Autodesk Inventor part; units mm, degrees
ref_plane "YZ Plane" through (0, 0, 0) normal (1, 0, 0) x (0, 1, 0)
ref_plane "XZ Plane" through (0, 0, 0) normal (0, 1, 0) x (-1, 0, 0)
ref_plane "XY Plane" through (0, 0, 0) normal (0, 0, 1) x (1, 0, 0)
sketch "Sketch1" plane through (0, 0, 0) normal (0, 0, 1) x (1, 0, 0)
  line L0 (-125.5, -122) -> (125.5, -122)
  line L1 (125.5, -122) -> (125.5, 122)
  line L2 (125.5, 122) -> (-125.5, 122)
  line L3 (-125.5, 122) -> (-125.5, -122)
  line L4 (-125.5, -122) -> (125.5, 122) construction
  line L5 (125.5, -122) -> (-125.5, 122) construction
  line L6 (125.5, 122) -> (47.5, 122)
  line L7 (47.5, 122) -> (47.5, 51)
  line L8 (47.5, 51) -> (125.5, 51)
  line L9 (125.5, 51) -> (125.5, 122)
  point P0 (0, 0)
  point P1 (125.5, 51)
  dimension "d0" = 251
  dimension "d1" = 244
  dimension "d6" = 78
  dimension "d7" = 71
extrude "Extrusion1" add sketch "Sketch1" along normal blind 7 contours L3 L2 L7 L8 L1 L0
sketch "Sketch2" plane through (0, 0, 7) normal (0, 0, 1) x (1, 0, 0)
  line L0 (-100, -100) -> (100, -100)
  line L1 (100, -100) -> (100, 100)
  line L2 (100, 100) -> (-100, 100)
  line L3 (-100, 100) -> (-100, -100)
  line L4 (-100, -100) -> (100, 100) construction
  line L5 (100, -100) -> (-100, 100) construction
  point P0 (0, 0)
  point P1 (0, 0)
  dimension "d4" = 200
  dimension "d5" = 200
sketch "Sketch3" plane through (0, 0, 7) normal (0, 0, 1) x (1, 0, 0)
  line L0 (-85.5721, 144.9839) -> (-125.5, 112)
  line L1 (-125.5, 122) -> (-125.5, -122)
  line L2 (-85.5721, 144.9839) -> (-17.6358, 144.9839) construction
  line L3 (125.5, -122) -> (125.5, 51)
  line L4 (125.5, 51) -> (47.5, 51)
  line L5 (47.5, 51) -> (47.5, 122)
  line L6 (47.5, 122) -> (-125.5, 122)
  line L7 (-125.5, 122) -> (-125.5, -122)
  line L8 (-125.5, -122) -> (125.5, -122)
  point P0 (0, 0)
  point P1 (-113.3947, 122)
  point P2 (-125.5, 122)
  dimension "d9" = 140.44
  dimension "d10" = 10
extrude "Extrusion2" cut sketch "Sketch3" against normal blind 10 contours L0 L1 L6
fillet "Fillet1" radius 5 2 edges at (-113.3947, 122, 3.5) (-125.5, 112, 3.5)
chamfer "Chamfer1" distance 10 angle 45 1 edges at (47.5, 51, 3.5)
sketch "Sketch4" plane through (0, 0, 7) normal (0, 0, 1) x (1, 0, 0)
  line L0 (-125.5, 109.645) -> (-125.5, -122)
  line L1 (125.5, -122) -> (125.5, 51)
  line L2 (-125.5, -122) -> (125.5, -122)
  point P0 (0, 0)
  point P1 (-121, -114.5)
  point P2 (115.5, -114.5)
  point P3 (10, -114.5)
  point P4 (62.75, -114.5)
  dimension "d17" = 4.5
  dimension "d20" = 10
  dimension "d21" = 7.5
  dimension "d42" = 52.75
  dimension "d43" = 52.75
hole "Hole1" at (-121, -114.5, 7) at (115.5, -114.5, 7) at (62.75, -114.5, 7) direction (0, 0, -1) diameter 3 depth 15 countersink diameter 6 countersink angle 100
sketch "Sketch5" plane through (0, 0, 7) normal (0, 0, 1) x (1, 0, 0)
  line L0 (-96.82, 94.1) -> (85.02, 94.1)
  line L1 (85.02, 94.1) -> (85.02, -109.4)
  line L2 (85.02, -109.4) -> (-96.82, -109.4)
  line L3 (-96.82, -109.4) -> (-96.82, 94.1)
  line L4 (125.5, -122) -> (125.5, 51)
  line L5 (-125.5, 109.645) -> (-125.5, -122)
  line L6 (47.5, 122) -> (-111.5966, 122)
  line L7 (-125.5, -122) -> (125.5, -122)
  circle A0 centre (115.5, -114.5) radius 3
  circle A1 centre (-121, -114.5) radius 3
  arc A2 (-123.6844, 113.4998) -> (-125.5, 109.645) centre (-120.5, 109.645) ccw
  line L8 (-125.5, 109.645) -> (-125.5, -122)
  line L9 (-125.5, -122) -> (125.5, -122)
  line L10 (125.5, -122) -> (125.5, 51)
  line L11 (125.5, 51) -> (57.5, 51)
  line L12 (47.5, 61) -> (57.5, 51)
  line L13 (47.5, 61) -> (47.5, 122)
  line L14 (47.5, 122) -> (-111.5966, 122)
  arc A3 (-111.5966, 122) -> (-114.781, 120.8548) centre (-111.5966, 117) ccw
  line L15 (-114.781, 120.8548) -> (-123.6844, 113.4998)
  point P0 (0, 0)
  point P1 (47.5, 94.1)
  point P2 (-111.5966, 122)
  point P3 (85.02, 51)
  dimension "d29" = 40.48
  dimension "d30" = 28.68
  dimension "d31" = 27.9
  dimension "d32" = 12.6
extrude "Extrusion3" cut sketch "Sketch5" against normal blind 1 contours L3 L2 L1 L11 L4 L7 L5 A2 L15 A3 L6 L13 L0 | A0 | A1
sketch "Sketch6" plane through (0, 0, 6) normal (0, 0, 1) x (1, 0, 0)
  circle A0 centre (115.5, -114.5) radius 1.8082
  circle A1 centre (-121, -114.5) radius 1.8082
  line L0 (47.5, 94.1) -> (-96.82, 94.1)
  line L1 (47.5, 122) -> (47.5, 94.1)
  line L2 (-111.5966, 122) -> (47.5, 122)
  arc A2 (-111.5966, 122) -> (-114.781, 120.8548) centre (-111.5966, 117) ccw
  line L3 (-123.6844, 113.4998) -> (-114.781, 120.8548)
  arc A3 (-123.6844, 113.4998) -> (-125.5, 109.645) centre (-120.5, 109.645) ccw
  line L4 (-125.5, -122) -> (-125.5, 109.645)
  line L5 (125.5, -122) -> (-125.5, -122)
  line L6 (125.5, 51) -> (125.5, -122)
  line L7 (85.02, 51) -> (125.5, 51)
  line L8 (85.02, -109.4) -> (85.02, 51)
  line L9 (-96.82, -109.4) -> (85.02, -109.4)
  line L10 (-96.82, 94.1) -> (-96.82, -109.4)
  circle A4 centre (62.75, -114.5) radius 1.8082
  circle A5 centre (115.5, -114.5) radius 1.8082
  circle A6 centre (-121, -114.5) radius 1.8082
  line L11 (47.5, 94.1) -> (-96.82, 94.1)
  line L12 (47.5, 122) -> (47.5, 94.1)
  line L13 (-111.5966, 122) -> (47.5, 122)
  arc A7 (-111.5966, 122) -> (-114.781, 120.8548) centre (-111.5966, 117) ccw
  line L14 (-123.6844, 113.4998) -> (-114.781, 120.8548)
  arc A8 (-123.6844, 113.4998) -> (-125.5, 109.645) centre (-120.5, 109.645) ccw
  line L15 (-125.5, -122) -> (-125.5, 109.645)
  line L16 (125.5, -122) -> (-125.5, -122)
  line L17 (125.5, 51) -> (125.5, -122)
  line L18 (85.02, 51) -> (125.5, 51)
  line L19 (85.02, -109.4) -> (85.02, 51)
  line L20 (-96.82, -109.4) -> (85.02, -109.4)
  line L21 (-96.82, 94.1) -> (-96.82, -109.4)
  point P0 (0, 0)
hole "Hole2" at (-121, -114.5, 6) at (115.5, -114.5, 6) at (62.75, -114.5, 6) direction (0, 0, -1) diameter 3 depth 15 countersink diameter 6 countersink angle 100
sketch "Sketch7" plane through (0, 0, 6) normal (0, 0, 1) x (1, 0, 0)
  circle A0 centre (62.75, -114.5) radius 3
  circle A1 centre (115.5, -114.5) radius 3
  circle A2 centre (-121, -114.5) radius 3
  line L0 (47.5, 94.1) -> (-96.82, 94.1)
  line L1 (47.5, 122) -> (47.5, 94.1)
  line L2 (-111.5966, 122) -> (47.5, 122)
  arc A3 (-111.5966, 122) -> (-114.781, 120.8548) centre (-111.5966, 117) ccw
  line L3 (-123.6844, 113.4998) -> (-114.781, 120.8548)
  arc A4 (-123.6844, 113.4998) -> (-125.5, 109.645) centre (-120.5, 109.645) ccw
  line L4 (-125.5, -122) -> (-125.5, 109.645)
  line L5 (125.5, -122) -> (-125.5, -122)
  line L6 (125.5, 51) -> (125.5, -122)
  line L7 (85.02, 51) -> (125.5, 51)
  line L8 (85.02, -109.4) -> (85.02, 51)
  line L9 (-96.82, -109.4) -> (85.02, -109.4)
  line L10 (-96.82, 94.1) -> (-96.82, -109.4)
  point P0 (0, 0)
  point P1 (113.25, 34.75)
  point P2 (113.25, -5.75)
  point P3 (113.25, -46.25)
  point P4 (113.25, -86.75)
  point P5 (-113.25, -86)
  point P6 (-113.25, -44)
  point P7 (-113.25, -2)
  point P8 (-113.25, 40)
  point P9 (-113.25, 82)
  dimension "d44" = 12.25
  dimension "d45" = 35.25
  dimension "d46" = 40.5
  dimension "d47" = 40.5
  dimension "d48" = 40.5
  dimension "d56" = 36
  dimension "d57" = 42
  dimension "d58" = 42
  dimension "d59" = 42
  dimension "d60" = 42
  dimension "d61" = 12.25
hole "Hole3" at (113.25, 34.75, 6) at (113.25, -5.75, 6) at (113.25, -46.25, 6) at (113.25, -86.75, 6) at (-113.25, 82, 6) at (-113.25, 40, 6) at (-113.25, -2, 6) at (-113.25, -44, 6) at (-113.25, -86, 6) direction (0, 0, -1) diameter 3 depth 10 countersink diameter 6 countersink angle 100
sketch "Sketch8" plane through (0, 0, 0) normal (0, 0, -1) x (-1, 0, 0)
  circle A0 centre (113.25, -86) radius 1.5
  circle A1 centre (113.25, -44) radius 1.5
  circle A2 centre (113.25, -2) radius 1.5
  circle A3 centre (113.25, 40) radius 1.5
  circle A4 centre (113.25, 82) radius 1.5
  circle A5 centre (-113.25, -86.75) radius 1.5
  circle A6 centre (-113.25, -46.25) radius 1.5
  circle A7 centre (-113.25, -5.75) radius 1.5
  circle A8 centre (-113.25, 34.75) radius 1.5
  circle A9 centre (-62.75, -114.5) radius 1.5
  circle A10 centre (-115.5, -114.5) radius 1.5
  circle A11 centre (121, -114.5) radius 1.5
  arc A12 (125.5, 109.645) -> (123.6844, 113.4998) centre (120.5, 109.645) ccw
  line L0 (123.6844, 113.4998) -> (114.781, 120.8548)
  arc A13 (114.781, 120.8548) -> (111.5966, 122) centre (111.5966, 117) ccw
  line L1 (-47.5, 122) -> (111.5966, 122)
  line L2 (-47.5, 61) -> (-47.5, 122)
  line L3 (-57.5, 51) -> (-47.5, 61)
  line L4 (-125.5, 51) -> (-57.5, 51)
  line L5 (-125.5, -122) -> (-125.5, 51)
  line L6 (125.5, -122) -> (-125.5, -122)
  line L7 (125.5, 109.645) -> (125.5, -122)
  line L8 (108.75, 122) -> (108.75, -122)
  line L9 (8.75, 122) -> (8.75, -122)
  line L10 (108.75, -112) -> (8.75, -112)
  point P0 (0, 0)
  dimension "d62" = 4.5
  dimension "d63" = 100
  dimension "d66" = 10
extrude "Extrusion4" cut sketch "Sketch8" against normal blind 3.25 contours L10 L9 L1 L8
fillet "Fillet2" radius 5 2 edges at (47.5, 61, 3.5) (57.5, 51, 3.5)
sketch "Sketch9" plane through (0, 0, 6) normal (0, 0, 1) x (1, 0, 0)
  circle A0 centre (-113.25, -86) radius 3
  circle A1 centre (-113.25, -44) radius 3
  circle A2 centre (-113.25, -2) radius 3
  circle A3 centre (-113.25, 40) radius 3
  circle A4 centre (-113.25, 82) radius 3
  circle A5 centre (113.25, -86.75) radius 3
  circle A6 centre (113.25, -46.25) radius 3
  circle A7 centre (113.25, -5.75) radius 3
  circle A8 centre (113.25, 34.75) radius 3
  circle A9 centre (62.75, -114.5) radius 3
  circle A10 centre (115.5, -114.5) radius 3
  circle A11 centre (-121, -114.5) radius 3
  line L0 (47.5, 94.1) -> (-96.82, 94.1)
  line L1 (47.5, 122) -> (47.5, 94.1)
  line L2 (-111.5966, 122) -> (47.5, 122)
  arc A12 (-111.5966, 122) -> (-114.781, 120.8548) centre (-111.5966, 117) ccw
  line L3 (-123.6844, 113.4998) -> (-114.781, 120.8548)
  arc A13 (-123.6844, 113.4998) -> (-125.5, 109.645) centre (-120.5, 109.645) ccw
  line L4 (-125.5, -122) -> (-125.5, 109.645)
  line L5 (125.5, -122) -> (-125.5, -122)
  line L6 (125.5, 51) -> (125.5, -122)
  line L7 (85.02, 51) -> (125.5, 51)
  line L8 (85.02, -109.4) -> (85.02, 51)
  line L9 (-96.82, -109.4) -> (85.02, -109.4)
  line L10 (-96.82, 94.1) -> (-96.82, -109.4)
  line L11 (47.5, 116) -> (-120.6579, 116)
  point P0 (0, 0)
  dimension "d68" = 6
extrude "Extrusion5" cut sketch "Sketch9" against normal through all contours L11 L3 A12 L2 L1
fillet "Fillet3" radius 5 1 edges at (-120.6579, 116, 3)
sketch "Sketch10" plane through (0, 0, 0) normal (0, 0, -1) x (-1, 0, 0)
  arc A0 (122.0442, 114.8548) -> (118.8598, 116) centre (118.8598, 111) ccw
  line L0 (118.8598, 116) -> (108.75, 116)
  line L1 (108.75, 116) -> (108.75, -112)
  line L2 (108.75, -112) -> (8.75, -112)
  line L3 (8.75, -112) -> (8.75, 116)
  line L4 (8.75, 116) -> (-47.5, 116)
  line L5 (-47.5, 63.0711) -> (-47.5, 116)
  arc A1 (-48.9645, 59.5355) -> (-47.5, 63.0711) centre (-52.5, 63.0711) ccw
  line L6 (-56.0355, 52.4645) -> (-48.9645, 59.5355)
  arc A2 (-59.5711, 51) -> (-56.0355, 52.4645) centre (-59.5711, 56) ccw
  line L7 (-125.5, 51) -> (-59.5711, 51)
  line L8 (-125.5, -122) -> (-125.5, 51)
  line L9 (125.5, -122) -> (-125.5, -122)
  line L10 (125.5, 109.645) -> (125.5, -122)
  arc A3 (125.5, 109.645) -> (123.6844, 113.4998) centre (120.5, 109.645) ccw
  line L11 (123.6844, 113.4998) -> (122.0442, 114.8548)
  circle A4 centre (121, -114.5) radius 1.5
  circle A5 centre (-115.5, -114.5) radius 1.5
  circle A6 centre (-62.75, -114.5) radius 1.5
  circle A7 centre (-113.25, 34.75) radius 1.5
  circle A8 centre (-113.25, -5.75) radius 1.5
  circle A9 centre (-113.25, -46.25) radius 1.5
  circle A10 centre (-113.25, -86.75) radius 1.5
  circle A11 centre (113.25, 82) radius 1.5
  circle A12 centre (113.25, 40) radius 1.5
  circle A13 centre (113.25, -2) radius 1.5
  circle A14 centre (113.25, -44) radius 1.5
  circle A15 centre (113.25, -86) radius 1.5
  line L12 (-123, 51) -> (-123, -122)
  line L13 (123, 114.0652) -> (123, -122)
  point P0 (0, 0)
  dimension "d72" = 2.5
  dimension "d73" = 2.5
extrude "Extrusion6" cut sketch "Sketch10" against normal through all contours L11 A3 L10 L9 L13 | L9 L8 L7 L12
fillet "Fillet4" radius 5 3 edges at (-123, 114.0652, 3) (-123, -122, 3) (123, -122, 3)
equation "\"d73\" = d72"
properties part number "ElectronicsBase" material "ABS Plastic"
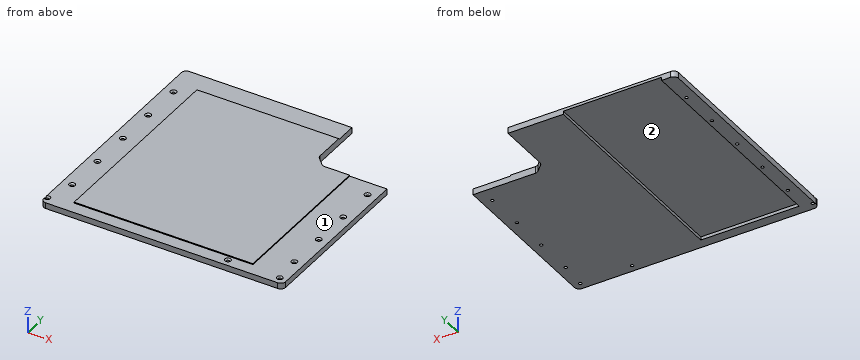
Could you check a few things on this model? Use its own coordinates, in mm. Face numbers are marked on the shaded views. Round coordinates to 2 decimals unless told otherwise and drop trailing zeros. Write each loop counter-clockwise with the first axis right and the second up, starting at its lowest first coordinate (ties: lowest second). Pieces come first, ordered by that corner, then holes. Notation, with made-up numbers: (79, -0.75) - (107, -0.75) arc R15 cw to (107, 8.25) - close; hole circle Ø5 at (46.25, 65.25). An arc over 180 degrees is marked (long way). Use a Markdown table: item, result.
Q1. For pin 1 (2 mm diameter, centred on y = 102, z = 5, fed in from +X); pin 2 (3.5 mm diameter, centred on x = 97, z = 2.5, fed in from +Y); pin 3 (6 mm diameter, centred on x = 97.5, y = -44, fed in from +Z), each with a flat end and sliding along its axis, tell me the tip position at first contact or that it passes through.
Output values:
| item | result |
|---|---|
| pin 1 | x = 47.5 |
| pin 2 | y = 51 |
| pin 3 | z = 6 |
Q2. I want a section at A-A (x = 3). List the corners of the cut face in (y, z) for me.
Output values:
| item | result |
|---|---|
| outline | (-122, 0) - (116, 0) - (116, 6) - (94.1, 6) - (94.1, 7) - (-109.4, 7) - (-109.4, 6) - (-122, 6) - close |
Q3. I want a section at D-D (x = -77). List the corners of the cut face in (y, z) for me, plus the area to 4 significant figures.
Output values:
| item | result |
|---|---|
| outline | (-122, 0) - (-112, 0) - (-112, 3.25) - (116, 3.25) - (116, 6) - (94.1, 6) - (94.1, 7) - (-109.4, 7) - (-109.4, 6) - (-122, 6) - close |
| area | 890.5 mm2 |
Q4. I want a section at C-C (z = 1.25). Count the separate pieces of the cut face and the enclosed holes in it, plus the area to 3 significant figures.
Output values:
| item | result |
|---|---|
| separate pieces | 1 |
| enclosed holes | 12 |
| area | 30,800 mm2 |
Q5. Thinking about a two-plate mould opening in X: for the marked faces 1 and 2, which applies, released by +X, released by -X, zero draft, split by the parting line, or undercut?
Output values:
| item | result |
|---|---|
| face 1 | zero draft |
| face 2 | undercut |
Q6. I want a section at B-B (y = -21). List the corners of the cut face in (x, z) for me, plus the area to 3 significant figures.
Output values:
| item | result |
|---|---|
| outline | (-123, 0) - (-108.75, 0) - (-108.75, 3.25) - (-8.75, 3.25) - (-8.75, 0) - (123, 0) - (123, 6) - (85.02, 6) - (85.02, 7) - (-96.82, 7) - (-96.82, 6) - (-123, 6) - close |
| area | 1,330 mm2 |
Q7. Please list where these lines run through material, in increasing order: L1, parallel to Y at x = 113.25, z = 1.55; L2, parallel to Y at x = -113.25, z = 1.1; L3, parallel to X at y = 20.5, z = 2.5.
Output values:
| item | result |
|---|---|
| L1 | -122 to -88.25, -85.25 to -47.75, -44.75 to -7.25, -4.25 to 33.25, 36.25 to 51 |
| L2 | -122 to -87.5, -84.5 to -45.5, -42.5 to -3.5, -0.5 to 38.5, 41.5 to 80.5, 83.5 to 116 |
| L3 | -123 to -108.75, -8.75 to 123 |
